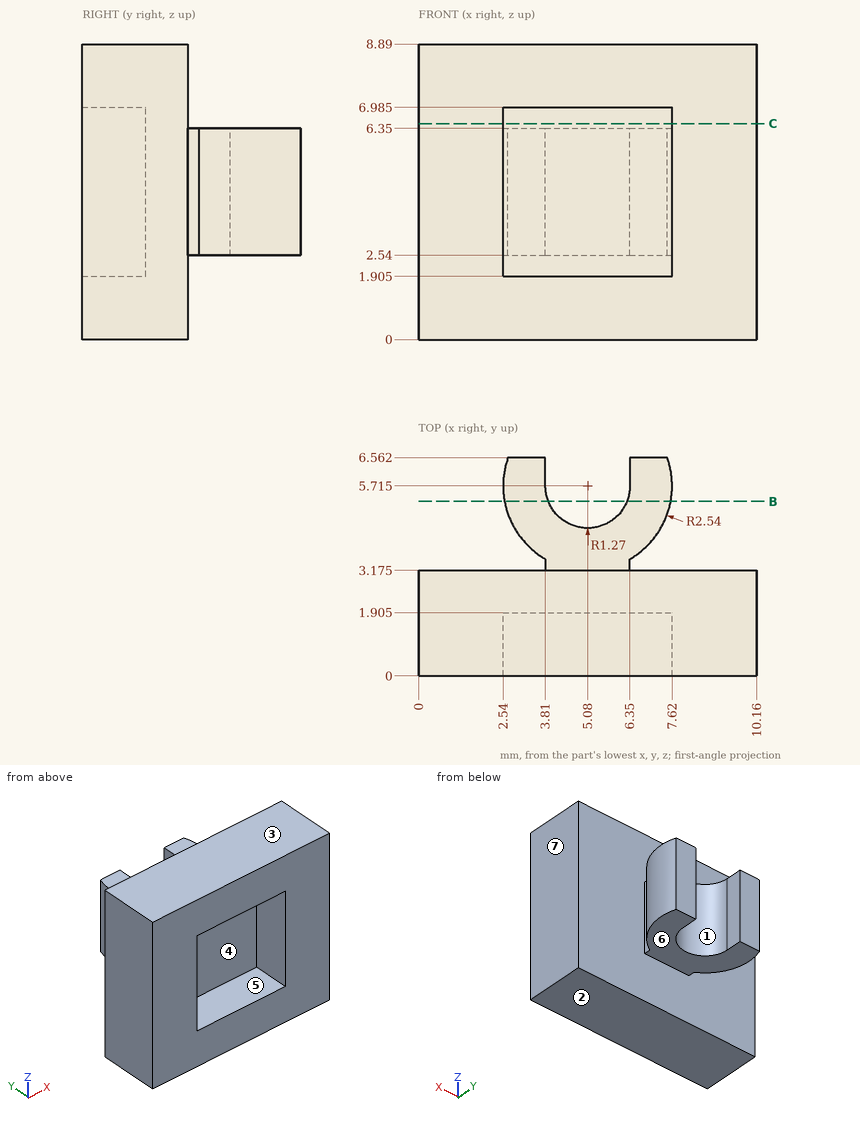
Answer from the drawing. Dimensions are ordinates in mm from the lowest x, y and z of the part. A direction names the side the tool comes from. Coordinates: 2 decimals unless noted, no trailing zeros. Loops run counter-clockwise (first coordinate to the right, second up) from the corner with the lowest first, then second, coordinate; pieces in that order, holes last.
Q1. The part is cut by section B-B on y = 5.25. Write down the section's boundary in (x, z), and give its area (3 significant figures).
Q2. Each of these flat-tipped pins is pushed along its axis until it touches: pin 1 Ø1.5 at (x, z) = (5, 5) entering from -Y (3 decimals); pin 2 Ø1 at (x, y) = (4, 4.5) entering from +Z; pin 3 Ø1 at (x, y) = (4, 5.5) entering from -Z. Where does it stop, or does it pass through?
Q3. The mould has two halves that part along Z. Classify the marked faces 1, 2, 3 and 4: +Z half, -Z half, draft (parallel to the pull), parting line (faces both ways), or undercut.
Q4. The part is cut by section C-C on z = 6.5. Write down the section's boundary in (x, y) (1 decimal), and give its area (3 significant figures).
Q5. Consider probe 1 along Z at (x, y) = (2.75, 5.5); probe 2 along Y at (x, z) = (2.25, 1) (1 decimal); probe 3 along Y at (x, z) = (3.75, 6.5) (1 decimal). Determine where each line is inside the solid, lowest interval first.
Q6. Which of the six approach directions +Z, -Z, +X, -X, +Y, -Y give full straight-line access (tool end or side, diameter ignored) to the marked faces 5, 6 and 7?
Results below:
1. outline: (2.58, 2.54) - (3.9, 2.54) - (3.9, 6.35) - (2.58, 6.35) - close; (6.26, 2.54) - (7.58, 2.54) - (7.58, 6.35) - (6.26, 6.35) - close
1. area: 10.0 mm2
2. pin 1: stops at y = 1.905
2. pin 2: stops at z = 6.35
2. pin 3: stops at z = 2.54
3. face 1: draft
3. face 2: -Z half
3. face 3: +Z half
3. face 4: undercut
4. outline: (0, 0) - (2.5, 0) - (2.5, 1.9) - (7.6, 1.9) - (7.6, 0) - (10.2, 0) - (10.2, 3.2) - (0, 3.2) - close
4. area: 22.6 mm2
5. probe 1: z = 2.54 to 6.35
5. probe 2: y = 0 to 3.2
5. probe 3: y = 1.9 to 3.2
6. face 5: -Y
6. face 6: -Z, +X, -X, +Y
6. face 7: +Z, -Z, +X, +Y, -Y
